Build history of the part. All positions in model axes, mm. Face numbers are marked on the shaded views. A direction names the side the tool comes from. Coordinates: 2 decimals unless noted, no trailing zeros. Loops run counter-clockwise (first coordinate to the right, second up) from the corner with the lowest first, then second, coordinate; pieces in that order, holes last.
Item 1: Flat gauge pins, fed straight in: pin 1 (8.5 mm diameter, centred on x = 15, z = -8, fed in from -Y); pin 2 (5.5 mm diameter, centred on x = 17, z = -10.5, fed in from +Y). Where does each tip first touch, or does it go through?
Item 2: Cut at D-D (x = 4). List the corners of the cut face in (y, z).
Item 3: Mould opens along Z. For the marked faces 3, 4, 5 and 6 say: released by +Z, released by -Z, zero draft, split by the parting line, or undercut.
Item 4: Cut at B-B (z = -10.75). Count the separate pieces of the cut face and the enclosed holes in it, and give its area (3 significant figures).
Item 5: Drill centre lines: line 1 along X through (y, z) = (5.2, -8); line 2 along X through (y, z) = (1.85, -8); line 3 along Z through (x, y) = (45, 1.25). Where is each one in solid material? Low to high.
Item 6: Cut at C-C (y = 5.25). List the corners of the cut face in (x, z).
Item 7: Cut at A-A (x = 45). List the corners of the cut face in (y, z), and give its area (3 significant figures).
Item 8: 3-axis set-ups, long thin cutter, end or side, ignore diameter. For the marked faces 1 and 2: which of +Z, -Z, +X, -X, +Y, -Y reach the whole face in a straight line?
from build123d import *

# Parameters (mm, degrees)
SKETCH_1_W          = 60
SKETCH_1_H          = 16
EXTRUDE_1_DEPTH     = 8.5
SKETCH_2_R          = 5.5
CUT_EXTRUDE_1_DEPTH = 4.5
EXTRUDE_2_DEPTH     = 1.5
SKETCH_3_R          = 3.3
CUT_EXTRUDE_2_DEPTH = 5
CHAMFER_1_SIZE      = 1.5


with BuildPart() as part:
    # 草图1 → 凸台-拉伸1 (new body)
    with BuildSketch(Plane(origin=(0, 0, 0), x_dir=(1, 0, 0), z_dir=(0, 1, 0))):
        with Locations((30, 8)):
            Rectangle(SKETCH_1_W, SKETCH_1_H)
    extrude(amount=EXTRUDE_1_DEPTH)

    # 草图2 → 切除-拉伸1 (cut)
    with BuildSketch(Plane(origin=(0, 8.5, 0), x_dir=(1, 0, 0), z_dir=(0, 1, 0))):
        with Locations((15, 8)):
            Circle(SKETCH_2_R)
        with Locations((45, 8)):
            Circle(SKETCH_2_R)
    extrude(amount=-CUT_EXTRUDE_1_DEPTH, mode=Mode.SUBTRACT)

    # 草图2<3> → 凸台-拉伸2 (add)
    with BuildSketch(Plane(origin=(0, 8.5, 0), x_dir=(1, 0, 0), z_dir=(0, 1, 0))):
        Polygon((0, 13.100505063), (0, 0), (13.100505063, 0), align=None)
        Polygon((16.899494937, 16), (32.899494937, 0), (43.100505063, 0), (27.100505063, 16), align=None)
        Polygon((46.899494937, 16), (60, 2.899494937), (60, 16), align=None)
    extrude(amount=EXTRUDE_2_DEPTH)

    # 草图3 → 切除-拉伸2 (cut, through all)
    with BuildSketch(Plane(origin=(0, 4, 0), x_dir=(1, 0, 0), z_dir=(0, 1, 0))):
        with Locations((15, 8)):
            Circle(SKETCH_3_R)
        with Locations((45, 8)):
            Circle(SKETCH_3_R)
    extrude(amount=-CUT_EXTRUDE_2_DEPTH, mode=Mode.SUBTRACT)

    # 倒角1
    chamfer_1_edges = [part.edges().sort_by_distance(p)[0] for p in [
        (6.550252532, 10, 0),
        (0, 10, -6.550252532),
        (22, 10, -16),
        (38, 10, 0),
        (60, 10, -9.449747468),
        (53.449747468, 10, -16),
    ]]
    chamfer(chamfer_1_edges, length=CHAMFER_1_SIZE)


solid = part.part
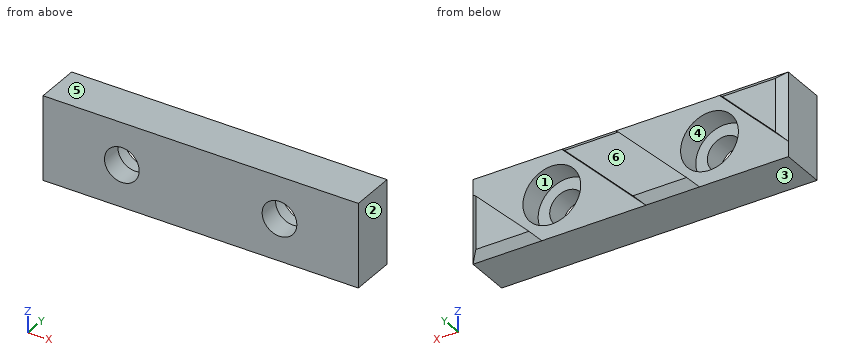
Filled sheet:
1. pin 1: stops at y = 0
1. pin 2: stops at y = 8.5
2. outline: (0, -16) - (8.5, -16) - (8.5, -9.1) - (10, -9.1) - (10, -1.5) - (8.5, 0) - (0, 0) - close
3. face 3: released by -Z
3. face 4: undercut
3. face 5: released by +Z
3. face 6: zero draft
4. separate pieces: 3
4. enclosed holes: 0
4. area: 423 mm2
5. line 1: x = 0 to 9.5, 20.5 to 39.5, 50.5 to 60
5. line 2: x = 0 to 11.7, 18.3 to 41.7, 48.3 to 60
5. line 3: z = -16 to -11.3, -4.7 to 0
6. outline: (0, -16) - (60, -16) - (60, 0) - (0, 0) - close; hole circle Ø11 at (15, -8); hole circle Ø11 at (45, -8)
7. outline: (0, -16) - (8.5, -16) - (8.5, -13.5) - (4, -13.5) - (4, -11.3) - (0, -11.3) - close; (0, -4.7) - (4, -4.7) - (4, -2.5) - (8.5, -2.5) - (8.5, 0) - (0, 0) - close
7. area: 60.1 mm2
8. face 1: +Y
8. face 2: +Z, -Z, +X, +Y, -Y
